Print and shaded views of the part. All mm, measured from the part's lowest x, y and z. A direction names the side the tool comes from. Round coordinates to 2 decimals unless told otherwise and drop trailing zeros. Order: outer loops, then holes, each group sorted by start corner. A loop starts at its lowest first (then second) coordinate and runs counter-clockwise, first axis right, second up. Notation, with made-up numbers: M 71,17 L 120,17 A22 ccw 120,32 Z; hole C 89.25,62.5 d10. An arc over 180 degrees is marked long. Use CSV: the item, a comma, the result in double quotes.
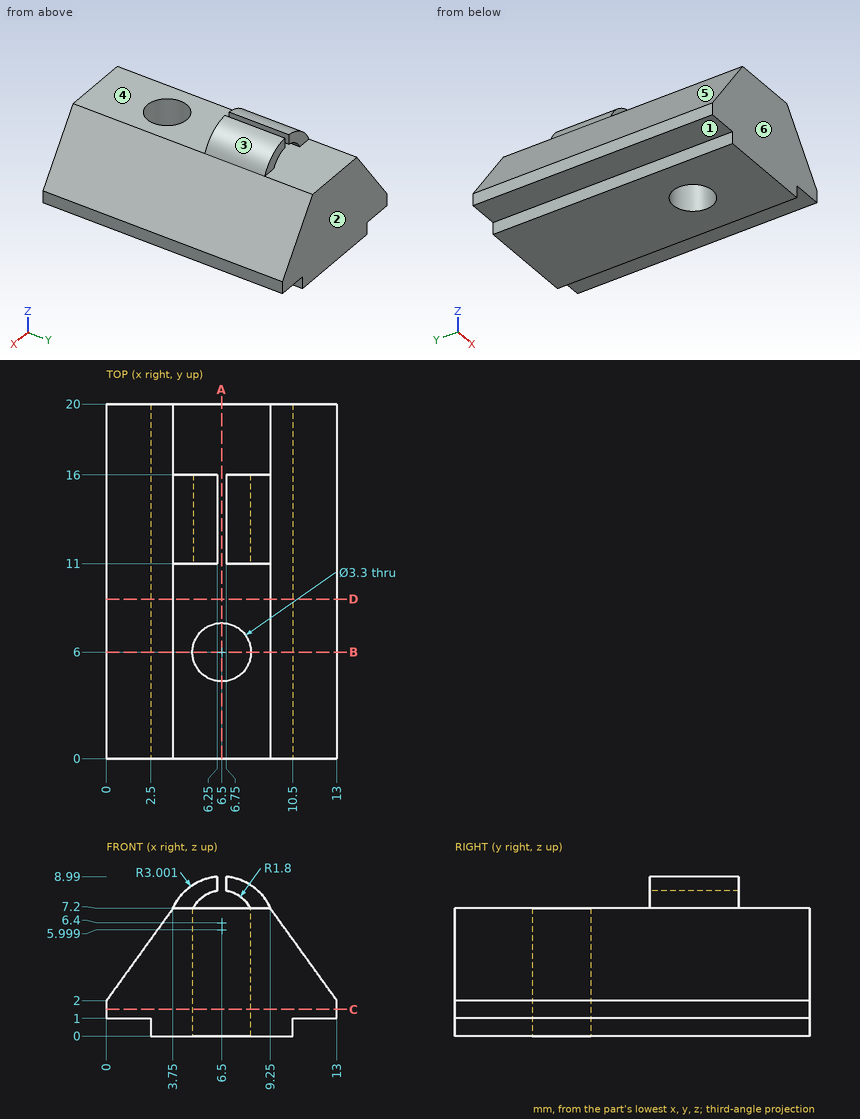
(1) Cut at A-A, the plane x = 6.5. Give the cut face in (y, z), and give its area (3 significant figures).
Answer block:
outline,"M 0,0 L 4.35,0 L 4.35,7.2 L 0,7.2 Z; M 7.65,0 L 20,0 L 20,7.2 L 7.65,7.2 Z"
area,"120 mm²"
(2) Wall check: line 1 (Y direction, x = 6.5, z = 4.25); line 2 (Z direction, x = 8, y = 3.25); line 3 (X direction, y = 15, z = 7.5) (1 decimal). Give the ranges that are in metal, low to high. Write a range as from..to.
Answer block:
line 1,"y = 0..4.35, 7.65..20"
line 2,"z = 0..7.2"
line 3,"x = 3.9..5.1, 7.9..9.1"
(3) Two-plate mould, pull along X, no slides. Class the marked faces 3, 4, 5 and 6: released by +X, released by -X, zero draft, split by the parting line, or undercut.
Answer block:
face 3,"released by +X"
face 4,"undercut"
face 5,"released by -X"
face 6,"zero draft"
(4) Cut at D-D, the plane y = 9. Give the cut face in (x, z), and give its area (3 significant figures).
Answer block:
outline,"M 0,1 L 2.5,1 L 2.5,0 L 10.5,0 L 10.5,1 L 13,1 L 13,2 L 9.25,7.2 L 3.75,7.2 L 0,2 Z"
area,"69.1 mm²"
(5) Tool access for the marked faces 1 and 2: list every direction of +Z, -Z, +X, -X, +Y, -Y with a clear straight run to the whole face (end or side of a thin tool).
Answer block:
face 1,"-Z, -X, +Y, -Y"
face 2,"+Z, -Z, +X, -X, +Y"
(6) Cut at B-B, the plane y = 6. Give the cut face in (x, z).
Answer block:
outline,"M 0,1 L 2.5,1 L 2.5,0 L 4.85,0 L 4.85,7.2 L 3.75,7.2 L 0,2 Z; M 8.15,0 L 10.5,0 L 10.5,1 L 13,1 L 13,2 L 9.25,7.2 L 8.15,7.2 Z"
(7) Drop flat-ended pins along their axis: pin 1 (1.4 mm diameter, centred on x = 8, z = 8, fed in from +Y); pin 2 (0.5 mm diameter, centred on y = 7, z = 0.5, fed in from -X); pin 3 (0.6 mm diameter, centred on y = 14, z = 8.5, fed in from +X). Give the stop position or say it passes through.
Answer block:
pin 1,"stops at y = 16"
pin 2,"stops at x = 2.5"
pin 3,"stops at x = 8.54"
(8) Cut at C-C, the plane z = 1.5. Give the cut face in (x, y).
Answer block:
outline,"M 0,0 L 13,0 L 13,20 L 0,20 Z; hole C 6.5,6 d3.3"
